Part model, mm, in its own coordinate system. Face numbers are marked on the shaded views. A direction names the side the tool comes from. Round coordinates to 2 decimals unless told otherwise and drop trailing zeros. Loops run counter-clockwise (first coordinate to the right, second up) from the corner with the lowest first, then second, coordinate; pieces in that order, holes last. Notation, with made-up numbers: (-13.5, -28) - (-0.5, -28) arc R24 ccw to (-0.5, 0) - close; hole circle Ø10 at (7, 20). An arc over 180 degrees is marked (long way). Put each result on its own line as item: value.
from build123d import *

# Parameters (mm, degrees)
FILLET1_R    = 0.8
SKETCH3_W    = 0.74
SKETCH3_H    = 3
SKETCH4_W    = 0.74
SKETCH4_H    = 0.99570227
RECPAT_COUNT = 2
RECPAT_ANGLE = 90


with BuildPart() as part:
    # BodySke → Base-Revolve (revolve)
    with BuildSketch(Plane.XY):
        Polygon((0, 0), (0, 2.75), (0.4, 2.75), (1.65, 1.5), (8, 1.5), (8, 0), align=None)
    revolve(axis=Axis((-6.35, 0, 0), (1, 0, 0)))

    # Fillet1
    fillet1_edges = [part.edges().sort_by_distance(p)[0] for p in [
        (1.65, -1.5, 0),
    ]]
    fillet(fillet1_edges, radius=FILLET1_R)

    # Sketch3 → Recess section 0
    with BuildSketch(Plane.ZY):
        Rectangle(SKETCH3_W, SKETCH3_H)
    # Sketch4 → Recess section 1
    with BuildSketch(Plane.ZY.offset(-2.01)):
        Rectangle(SKETCH4_W, SKETCH4_H)
    recess = loft(mode=Mode.SUBTRACT)

    # RecPat: Recess ×2 about axis
    recpat_axis = Axis((0, 0, 0), (1, 0, 0))
    for i in range(1, RECPAT_COUNT):
        add(recess.rotate(recpat_axis, i * RECPAT_ANGLE / (RECPAT_COUNT - 1)), mode=Mode.SUBTRACT)

    # RecCorSke → RecessCore (revolve, cut)
    with BuildSketch(Plane.XY):
        Polygon((0, 0), (0, 0.696552892), (2.01, 0.556), (2.190655351, 0), align=None)
    revolve(axis=Axis((-3.175, 0, 0), (1, 0, 0)), mode=Mode.SUBTRACT)


solid = part.part
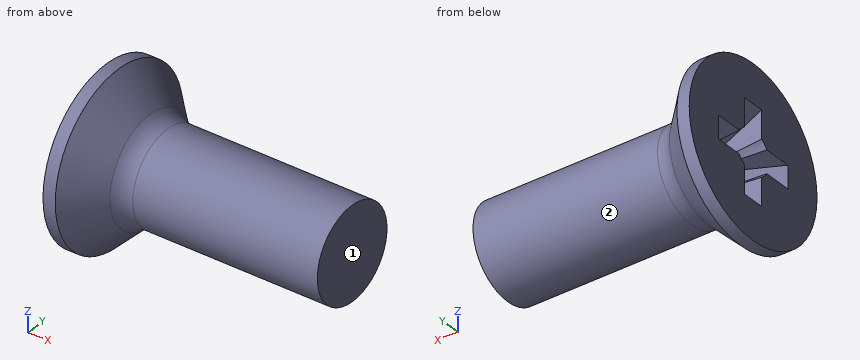
1. Band-saw the part on A-A (x = 3.25). List the corners of the cut face in (y, z).
A:
outline: circle Ø3 at (0, 0)
2. Pin check, flat tips, straight feed: P1, Ø3, axis at x = 3, y = -1.5, coming from the +Z side; P2, Ø3, axis at x = 4, z = -0.5, coming from the +Y side; P3, Ø2, axis at x = 5.5, y = 2, coming from the +Z side. Stop position of each tip, or through.
A:
P1: stops at z = 1.5
P2: stops at y = 1.5
P3: stops at z = 1.12
3. Probe line 1 along Y through (x, z) = (5, 0.95); line 2 along X through (y, z) = (-0.45, 0.2); line 3 along Z through (x, y) = (1, -1.25). List the from-to ranges inside material, lowest first. Write a range as [from, to].
A:
line 1: y = [-1.16, 1.16]
line 2: x = [2.03, 8]
line 3: z = [-1.75, 1.75]
4. Tool access for the marked faces 1 and 2: list every direction of +Z, -Z, +X, -X, +Y, -Y with a clear straight run to the whole face (end or side of a thin tool).
A:
face 1: +Z, -Z, +X, +Y, -Y
face 2: +X
